Geometry check sheet. Reference: the model listing, model coordinates, mm. Give positions to 0.01 mm unless a question says otherwise; leave off trailing zeros. Write each loop counter-clockwise with the first axis right and the second up, starting at its lowest first coordinate (ties: lowest second). Pieces come first, ordered by that corner, then holes. Notation, with made-up numbers: M 15.5,54 L 41.5,54 A14 ccw 41.5,64 Z; hole C -3.5,-6.5 d10. An arc over 180 degrees is marked long. One line per item, written item: value. Start each with the question number.
1. Cross-section at D-D on z = 1.5. Record the cut outline in (x, y) (3 decimals), then the cut area to 3 significant figures.
2. Cross-section at C-C on z = 0. Record the cut outline in (x, y), then the cut area to 4 significant figures.
3. Cross-section at A-A on x = 13. Record the cut outline in (y, z).
4. Scan lines: line 1 (X direction, y = 0.9, z = 2.25); line 2 (X direction, y = 0.95, z = -2). Record each from-to range of solid material in increasing order.
5. Cross-section at B-B on z = 3.5. Record the cut outline in (x, y).
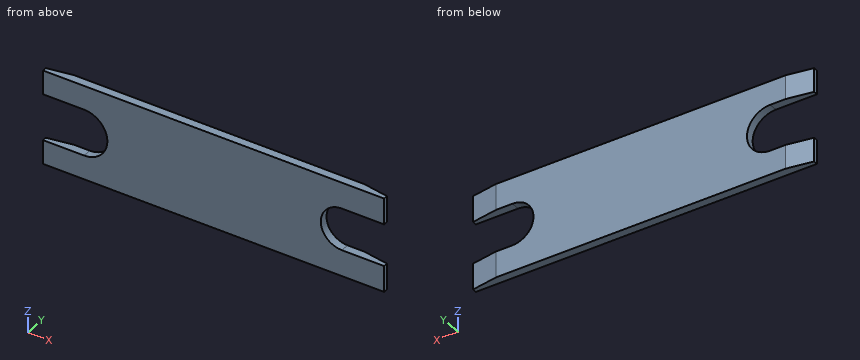
from build123d import *

# Parameters (mm, degrees)
SKETCH1_R           = 2.7
SKETCH1_R_2         = 2.45
BOSS_EXTRUDE1_DEPTH = 1
SKETCH2_W           = 5.5
SKETCH2_H           = 5.4
SKETCH2_H_2         = 4.9
CUT_EXTRUDE1_DEPTH  = 2
BOSS_EXTRUDE2_DEPTH = 1
CHAMFER1_SIZE       = 3
CHAMFER1_SIZE2      = 0.5


with BuildPart() as part:
    # Sketch1 → Boss-Extrude1 (new body)
    with BuildSketch(Plane(origin=(0, 0, 0), x_dir=(1, 0, 0), z_dir=(0, 1, 0))):
        with BuildLine():
            Line((-15, 5.5), (15, 5.5))
            ThreePointArc((15, 5.5), (20.5, 0), (15, -5.5))
            Line((15, -5.5), (-15, -5.5))
            ThreePointArc((-15, -5.5), (-20.5, 0), (-15, 5.5))
        make_face()
        with Locations((-15, 0)):
            Circle(SKETCH1_R, mode=Mode.SUBTRACT)
        with Locations((15, 0)):
            Circle(SKETCH1_R_2, mode=Mode.SUBTRACT)
    extrude(amount=BOSS_EXTRUDE1_DEPTH)

    # Sketch2 → Cut-Extrude1 (cut, through all)
    with BuildSketch(Plane(origin=(0, 1, 0), x_dir=(1, 0, 0), z_dir=(0, 1, 0))):
        with Locations((-17.75, 0)):
            Rectangle(SKETCH2_W, SKETCH2_H)
        with Locations((17.75, 0)):
            Rectangle(SKETCH2_W, SKETCH2_H_2)
    extrude(amount=-CUT_EXTRUDE1_DEPTH, mode=Mode.SUBTRACT)

    # Sketch3 → Boss-Extrude2 (add)
    with BuildSketch(Plane.XZ):
        with BuildLine():
            Line((-19.79165942, 2.7), (-19.79165942, 5.5))
            Line((-19.79165942, 5.5), (-15, 5.5))
            ThreePointArc((-15, 5.5), (-17.774887385, 4.748684028), (-19.79165942, 2.7))
        make_face()
        with BuildLine():
            Line((15, 5.5), (19.924175058, 5.5))
            Line((19.924175058, 5.5), (19.924175058, 2.45))
            ThreePointArc((19.924175058, 2.45), (17.896118092, 4.675735236), (15, 5.5))
        make_face()
        with BuildLine():
            Line((19.924175058, -2.45), (19.924175058, -5.5))
            Line((19.924175058, -5.5), (15, -5.5))
            ThreePointArc((15, -5.5), (17.896118092, -4.675735236), (19.924175058, -2.45))
        make_face()
        with BuildLine():
            Line((-15, -5.5), (-19.79165942, -5.5))
            Line((-19.79165942, -5.5), (-19.79165942, -2.7))
            ThreePointArc((-19.79165942, -2.7), (-17.774887385, -4.748684028), (-15, -5.5))
        make_face()
    extrude(amount=-BOSS_EXTRUDE2_DEPTH)

    # Chamfer1
    chamfer1_edges = [part.edges().sort_by_distance(p)[0] for p in [
        (19.924175058, 1, -3.975),
        (-19.79165942, 1, 4.1),
        (-19.79165942, 1, -4.1),
        (19.924175058, 1, 3.975),
    ]]
    chamfer1_side = [part.faces().sort_by_distance(p)[0] for p in [
        (0.231556515, 1, 0),
    ]]
    chamfer(chamfer1_edges, length=CHAMFER1_SIZE, length2=CHAMFER1_SIZE2, reference=chamfer1_side[0])


solid = part.part
Report:
1. outline: M -12.755,0 L 13.063,0 L 13.063,1 L -12.755,1 Z
1. area: 25.8 mm^2
2. outline: M -12.3,0 L 12.55,0 L 12.55,1 L -12.3,1 Z
2. area: 24.85 mm^2
3. outline: M 0,-5.5 L 1,-5.5 L 1,-1.42 L 0,-1.42 Z; M 0,1.42 L 1,1.42 L 1,5.5 L 0,5.5 Z
4. line 1: x = -13.51 to 14.03
4. line 2: x = -13.19 to 13.58
5. outline: M -19.79,0 L 19.92,0 L 19.92,0.5 L 16.92,1 L -16.79,1 L -19.79,0.5 Z
